from build123d import *

# Parameters (mm, degrees)
CROQUIS1_W              = 455
CROQUIS1_H              = 409
SALIENTE_EXTRUIR1_DEPTH = 1
CORTAR_EXTRUIR1_REACH   = 307.904
CROQUIS2_R              = 1.6
CORTAR_EXTRUIR2_REACH   = 307.904
CROQUIS3_R              = 5
CORTAR_EXTRUIR3_REACH   = 307.904
CROQUIS4_R              = 1.6


with BuildPart() as part:
    # Croquis1 → Saliente-Extruir1 (new body)
    with BuildSketch(Plane(origin=(0, 0, 0), x_dir=(1, 0, 0), z_dir=(0, 1, 0))):
        Rectangle(CROQUIS1_W, CROQUIS1_H)
    extrude(amount=SALIENTE_EXTRUIR1_DEPTH)

    # Croquis2 → Cortar-Extruir1 (cut, up to next)
    with BuildSketch(Plane.XZ, mode=Mode.PRIVATE) as cortar_extruir1_sk1:
        with Locations(Location((-215, 178.6, 0), (0, 0, 270))):
            Circle(CROQUIS2_R)
    cortar_extruir1_tool1 = extrude(cortar_extruir1_sk1.sketch, amount=-CORTAR_EXTRUIR1_REACH, mode=Mode.PRIVATE) & part.part
    # Croquis2 → Cortar-Extruir1 (cut, up to next)
    with BuildSketch(Plane.XZ, mode=Mode.PRIVATE) as cortar_extruir1_sk2:
        with Locations(Location((-215, -181.4, 0), (0, 0, 270))):
            Circle(CROQUIS2_R)
    cortar_extruir1_tool2 = extrude(cortar_extruir1_sk2.sketch, amount=-CORTAR_EXTRUIR1_REACH, mode=Mode.PRIVATE) & part.part
    # Croquis2 → Cortar-Extruir1 (cut, up to next)
    with BuildSketch(Plane.XZ, mode=Mode.PRIVATE) as cortar_extruir1_sk3:
        with Locations(Location((215, -181.4, 0), (0, 0, 270))):
            Circle(CROQUIS2_R)
    cortar_extruir1_tool3 = extrude(cortar_extruir1_sk3.sketch, amount=-CORTAR_EXTRUIR1_REACH, mode=Mode.PRIVATE) & part.part
    # Croquis2 → Cortar-Extruir1 (cut, up to next)
    with BuildSketch(Plane.XZ, mode=Mode.PRIVATE) as cortar_extruir1_sk4:
        with Locations(Location((215, 178.6, 0), (0, 0, 270))):
            Circle(CROQUIS2_R)
    cortar_extruir1_tool4 = extrude(cortar_extruir1_sk4.sketch, amount=-CORTAR_EXTRUIR1_REACH, mode=Mode.PRIVATE) & part.part
    # Croquis2 → Cortar-Extruir1 (cut, up to next)
    with BuildSketch(Plane.XZ, mode=Mode.PRIVATE) as cortar_extruir1_sk5:
        with Locations(Location((0, 31.25, 0), (0, 0, 270))):
            Circle(CROQUIS2_R)
    cortar_extruir1_tool5 = extrude(cortar_extruir1_sk5.sketch, amount=-CORTAR_EXTRUIR1_REACH, mode=Mode.PRIVATE) & part.part
    add(cortar_extruir1_tool1.solids().sort_by_distance((-215, 0, 178.6))[0], mode=Mode.SUBTRACT)
    add(cortar_extruir1_tool2.solids().sort_by_distance((-215, 0, -181.4))[0], mode=Mode.SUBTRACT)
    add(cortar_extruir1_tool3.solids().sort_by_distance((215, 0, -181.4))[0], mode=Mode.SUBTRACT)
    add(cortar_extruir1_tool4.solids().sort_by_distance((215, 0, 178.6))[0], mode=Mode.SUBTRACT)
    add(cortar_extruir1_tool5.solids().sort_by_distance((0, 0, 31.25))[0], mode=Mode.SUBTRACT)

    # Croquis3 → Cortar-Extruir2 (cut, up to next)
    with BuildSketch(Plane.XZ, mode=Mode.PRIVATE) as cortar_extruir2_sk1:
        with Locations(Location((-157.5, 38.6, 0), (0, 0, 270))):
            Circle(CROQUIS3_R)
    cortar_extruir2_tool1 = extrude(cortar_extruir2_sk1.sketch, amount=-CORTAR_EXTRUIR2_REACH, mode=Mode.PRIVATE) & part.part
    # Croquis3 → Cortar-Extruir2 (cut, up to next)
    with BuildSketch(Plane.XZ, mode=Mode.PRIVATE) as cortar_extruir2_sk2:
        with Locations(Location((-107.5, 38.6, 0), (0, 0, 270))):
            Circle(CROQUIS3_R)
    cortar_extruir2_tool2 = extrude(cortar_extruir2_sk2.sketch, amount=-CORTAR_EXTRUIR2_REACH, mode=Mode.PRIVATE) & part.part
    # Croquis3 → Cortar-Extruir2 (cut, up to next)
    with BuildSketch(Plane.XZ, mode=Mode.PRIVATE) as cortar_extruir2_sk3:
        with Locations(Location((-107.5, 188.6, 0), (0, 0, 270))):
            Circle(CROQUIS3_R)
    cortar_extruir2_tool3 = extrude(cortar_extruir2_sk3.sketch, amount=-CORTAR_EXTRUIR2_REACH, mode=Mode.PRIVATE) & part.part
    # Croquis3 → Cortar-Extruir2 (cut, up to next)
    with BuildSketch(Plane.XZ, mode=Mode.PRIVATE) as cortar_extruir2_sk4:
        with Locations(Location((-157.5, 188.6, 0), (0, 0, 270))):
            Circle(CROQUIS3_R)
    cortar_extruir2_tool4 = extrude(cortar_extruir2_sk4.sketch, amount=-CORTAR_EXTRUIR2_REACH, mode=Mode.PRIVATE) & part.part
    add(cortar_extruir2_tool1.solids().sort_by_distance((-157.5, 0, 38.6))[0], mode=Mode.SUBTRACT)
    add(cortar_extruir2_tool2.solids().sort_by_distance((-107.5, 0, 38.6))[0], mode=Mode.SUBTRACT)
    add(cortar_extruir2_tool3.solids().sort_by_distance((-107.5, 0, 188.6))[0], mode=Mode.SUBTRACT)
    add(cortar_extruir2_tool4.solids().sort_by_distance((-157.5, 0, 188.6))[0], mode=Mode.SUBTRACT)

    # Croquis4 → Cortar-Extruir3 (cut, up to next)
    with BuildSketch(Plane.XZ, mode=Mode.PRIVATE) as cortar_extruir3_sk1:
        with Locations(Location((-215, -1.4, 0), (0, 0, 270))):
            Circle(CROQUIS4_R)
    cortar_extruir3_tool1 = extrude(cortar_extruir3_sk1.sketch, amount=-CORTAR_EXTRUIR3_REACH, mode=Mode.PRIVATE) & part.part
    # Croquis4 → Cortar-Extruir3 (cut, up to next)
    with BuildSketch(Plane.XZ, mode=Mode.PRIVATE) as cortar_extruir3_sk2:
        with Locations(Location((215, -1.4, 0), (0, 0, 270))):
            Circle(CROQUIS4_R)
    cortar_extruir3_tool2 = extrude(cortar_extruir3_sk2.sketch, amount=-CORTAR_EXTRUIR3_REACH, mode=Mode.PRIVATE) & part.part
    # Croquis4 → Cortar-Extruir3 (cut, up to next)
    with BuildSketch(Plane.XZ, mode=Mode.PRIVATE) as cortar_extruir3_sk3:
        with Locations(Location((0, 188.6, 0), (0, 0, 270))):
            Circle(CROQUIS4_R)
    cortar_extruir3_tool3 = extrude(cortar_extruir3_sk3.sketch, amount=-CORTAR_EXTRUIR3_REACH, mode=Mode.PRIVATE) & part.part
    # Croquis4 → Cortar-Extruir3 (cut, up to next)
    with BuildSketch(Plane.XZ, mode=Mode.PRIVATE) as cortar_extruir3_sk4:
        with Locations(Location((30, -181.4, 0), (0, 0, 270))):
            Circle(CROQUIS4_R)
    cortar_extruir3_tool4 = extrude(cortar_extruir3_sk4.sketch, amount=-CORTAR_EXTRUIR3_REACH, mode=Mode.PRIVATE) & part.part
    add(cortar_extruir3_tool1.solids().sort_by_distance((-215, 0, -1.4))[0], mode=Mode.SUBTRACT)
    add(cortar_extruir3_tool2.solids().sort_by_distance((215, 0, -1.4))[0], mode=Mode.SUBTRACT)
    add(cortar_extruir3_tool3.solids().sort_by_distance((0, 0, 188.6))[0], mode=Mode.SUBTRACT)
    add(cortar_extruir3_tool4.solids().sort_by_distance((30, 0, -181.4))[0], mode=Mode.SUBTRACT)


solid = part.part
The listing builds one solid part. Answer for the finished solid, in the listing's coordinates (mm). Give positions to 0.01 mm unless a question says otherwise; leave off trailing zeros. Write each loop counter-clockwise with the first axis right and the second up, starting at its lowest first coordinate (ties: lowest second). Pieces come first, ordered by that corner, then holes.
Item 1: Section B-B, the plane z = 38.6 is taken. Write down the section's boundary in (x, y).
Item 2: Determine the mould class of faces 1 (the cylindrical face through (-152.543, 0.493, 39.251)), 2 (the flat face through (-3, 0, -3)) for opening direction Z: released by +Z, released by -Z, zero draft, split by the parting line, or undercut.
Item 3: Find the intervals of material crossed by line 1 along Z through (x, y) = (215, 0.5); line 2 along X through (y, z) = (0.6, -181.4); line 3 along X through (y, z) = (0.2, 178.6), in increasing order.
Item 4: Flat-ended cylindrical pins translate along their axes: P1, Ø10, axis at x = 179.5, z = 94, coming from the -Y side; P2, Ø3, axis at x = -215, z = -1.4, coming from the +Y side. Find the tip coordinate at first contact, or state that the pin passes through.
Item 5: Section A-A, the plane x = -107.5 is taken. Write down the section's boundary in (y, z).
Completed:
1. outline: (-227.5, 0) - (-162.5, 0) - (-162.5, 1) - (-227.5, 1) - close; (-152.5, 0) - (-112.5, 0) - (-112.5, 1) - (-152.5, 1) - close; (-102.5, 0) - (227.5, 0) - (227.5, 1) - (-102.5, 1) - close
2. face 1: undercut
2. face 2: zero draft
3. line 1: z = -204.5 to -183, -179.8 to -3, 0.2 to 177, 180.2 to 204.5
3. line 2: x = -227.5 to -216.6, -213.4 to 28.4, 31.6 to 213.4, 216.6 to 227.5
3. line 3: x = -227.5 to -216.6, -213.4 to 213.4, 216.6 to 227.5
4. P1: stops at y = 0
4. P2: passes through
5. outline: (0, -204.5) - (1, -204.5) - (1, 33.6) - (0, 33.6) - close; (0, 43.6) - (1, 43.6) - (1, 183.6) - (0, 183.6) - close; (0, 193.6) - (1, 193.6) - (1, 204.5) - (0, 204.5) - close
